For this review, take the finished solid that the model builds, in its own axes (mm). Face numbers are marked on the shaded views. A direction names the side the tool comes from. Coordinates: 2 decimals unless noted, no trailing zeros. Loops run counter-clockwise (first coordinate to the right, second up) from the corner with the lowest first, then second, coordinate; pieces in that order, holes last. Notation, with made-up numbers: (-4, 65) - (47, 65) arc R25 ccw to (47, 84) - close; hole circle Ø6 at (-17, 26.25). An arc over 180 degrees is marked (long way). Use one line per item in the form item = value. Start each with the question number.
1. Add section A-A on z = -35. Give the boundary of the cut face in (x, y).
2. For pin 1 Ø10 at (x, y) = (124.5, -20) entering from -Z; pin 2 Ø12.5 at (y, z) = (-15, 22) entering from +X; pin 3 Ø7.5 at (x, y) = (20.5, -8.5) entering from +Z; pin 4 Ø8 at (x, y) = (-37.5, -15.5) entering from +Z, all flat-tipped, find the tip position at first contact; note any pin that passes through.
3. Draft analysis for pull direction X (two halves, no side actions). For the marked faces 5, 6, 7 and 8, state which applies: +X half, -X half, draft (parallel to the pull), parting line (faces both ways), or undercut.
4. Add section C-C on z = -5. Give the boundary of the cut face in (x, y), and give its area (3 significant figures).
5. Add section B-B on x = 86. Give the boundary of the cut face in (y, z).
6. Add section D-D on z = -20.5. Give the boundary of the cut face in (x, y).
7. To check wall thickness, follow probe 1 along Z at (x, y) = (76, -8.5); probe 2 along X at (y, z) = (-11.5, -5.5); probe 3 along X at (y, z) = (-5.5, -26). State the ranges of each line that lie inside material, in increasing order.
8. Machinability: for the marked faces 1, 2, 3 and 4, which of the approach directions +Z, -Z, +X, -X, +Y, -Y give a long, thin tool a straight path to every point of the face, cutting with its end or side? Answer none if there is none.
```python
from build123d import *

# Parameters (mm, degrees)
F1_DEPTH = 25.4


with BuildPart() as f1:
    # F0 (on Front) → F1 (new body)
    with BuildSketch(Plane.XZ):
        Polygon((-58.56847018, 26.8058441579), (-58.56847018, 44.1696718335), (-75.8564463832, 44.1696718335), (-87.0612412691, 22.8805579245), (-98.826281338, 44.1696718335), (-116.1657199264, 44.1696718335), (-116.1657199264, -44.1696718335), (-97.4510317668, -44.1696718335), (-97.4510317668, 8.7780756876), (-87.0612412691, -2.158543095), (-75.5490139127, 8.7780756876), (-75.5490139127, -44.1696718335), (-58.56847018, -44.1696718335), align=None)
        Polygon((-7.5672003441, 26.8058441579), (-7.5672003441, 44.1696718335), (-16.0395050349, 44.1696718335), (-32.1926623583, 26.0362979025), (-50.0853913032, 44.1696718335), (-58.56847018, 44.1696718335), (-58.56847018, 26.8058441579), (-41.1093979278, 9.8758367822), (-41.1093979278, -44.1696718335), (-23.9841751754, -44.1696718335), (-23.9841751754, 9.8758367822), align=None)
        Polygon((9.3628074974, -29.6275112778), (9.3628074974, 44.1696718335), (-7.5672003441, 44.1696718335), (-7.5672003441, 26.8058441579), (-7.5672003441, -44.1696718335), (40.4011495411, -44.1696718335), (40.4011495411, -29.6275112778), align=None)
        Polygon((116.1657199264, 44.110127064), (116.1657199264, 44.1696718335), (40.4011495411, 44.1696718335), (40.4011495411, -29.6275112778), (40.4011495411, -44.1696718335), (116.1657199264, -44.1696718335), (116.1657199264, -44.110127064), (100.1692116261, -44.110127064), (100.1692116261, -25.7797837257), (63.4875297546, -25.7797837257), (63.4875297546, 5.258561112), (79.1349560022, 5.258561112), (79.1349560022, 15.0061408058), (63.4875297546, 15.0061408058), (63.4875297546, 26.5493281186), (100.1692116261, 26.5493281186), (100.1692116261, 44.110127064), align=None)
        Polygon((157.1156084538, 44.110127064), (116.1657199264, 44.110127064), (116.1657199264, -10.1323537529), (135.5683207512, -10.1323537529), (135.5683207512, -26.8058460206), (121.2034597993, -26.8058460206), (121.2034597993, -12.4409906566), (116.1657199264, -12.4409906566), (116.1657199264, -44.110127064), (157.1156084538, -44.110127064), (157.1156084538, 7.054167334), (119.920887053, 7.054167334), (119.920887053, 23.21462892), (157.1156084538, 23.21462892), align=None)
        Polygon((116.1657199264, -10.1323537529), (116.1657199264, 44.110127064), (100.1692116261, 44.110127064), (100.1692116261, 26.5493281186), (100.1692116261, -10.1323537529), align=None)
        Polygon((116.1657199264, -44.110127064), (116.1657199264, -12.4409906566), (100.1692116261, -12.4409906566), (100.1692116261, -25.7797837257), (100.1692116261, -44.110127064), align=None)
    extrude(amount=F1_DEPTH)


solid = f1.part
```
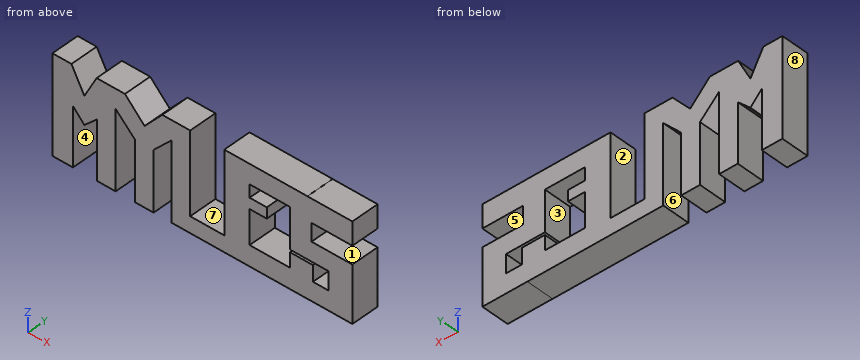
Conclusion:
q1.outline = (-116.17, -25.4) - (-97.45, -25.4) - (-97.45, 0) - (-116.17, 0) - close; (-75.55, -25.4) - (-58.57, -25.4) - (-58.57, 0) - (-75.55, 0) - close; (-41.11, -25.4) - (-23.98, -25.4) - (-23.98, 0) - (-41.11, 0) - close; (-7.57, -25.4) - (157.12, -25.4) - (157.12, 0) - (-7.57, 0) - close
q2.pin_1 = -44.11
q2.pin_2 = 157.12
q2.pin_3 = -29.63
q2.pin_4 = 35.47
q3.face_5 = draft
q3.face_6 = undercut
q3.face_7 = undercut
q3.face_8 = -X half
q4.outline = (-116.17, -25.4) - (-97.45, -25.4) - (-97.45, 0) - (-116.17, 0) - close; (-75.55, -25.4) - (-58.57, -25.4) - (-58.57, 0) - (-75.55, 0) - close; (-41.11, -25.4) - (-23.98, -25.4) - (-23.98, 0) - (-41.11, 0) - close; (-7.57, -25.4) - (9.36, -25.4) - (9.36, 0) - (-7.57, 0) - close; (40.4, -25.4) - (63.49, -25.4) - (63.49, 0) - (40.4, 0) - close; (100.17, -25.4) - (157.12, -25.4) - (157.12, 0) - (100.17, 0) - close
q4.area = 3,800 mm^2
q5.outline = (-25.4, -44.17) - (0, -44.17) - (0, -25.78) - (-25.4, -25.78) - close; (-25.4, 26.55) - (0, 26.55) - (0, 44.17) - (-25.4, 44.17) - close
q6.outline = (-116.17, -25.4) - (-97.45, -25.4) - (-97.45, 0) - (-116.17, 0) - close; (-75.55, -25.4) - (-58.57, -25.4) - (-58.57, 0) - (-75.55, 0) - close; (-41.11, -25.4) - (-23.98, -25.4) - (-23.98, 0) - (-41.11, 0) - close; (-7.57, -25.4) - (9.36, -25.4) - (9.36, 0) - (-7.57, 0) - close; (40.4, -25.4) - (63.49, -25.4) - (63.49, 0) - (40.4, 0) - close; (100.17, -25.4) - (121.2, -25.4) - (121.2, 0) - (100.17, 0) - close; (135.57, -25.4) - (157.12, -25.4) - (157.12, 0) - (135.57, 0) - close
q7.probe_1 = -44.17 to -25.78, 5.26 to 15.01, 26.55 to 44.17
q7.probe_2 = -116.17 to -97.45, -75.55 to -58.57, -41.11 to -23.98, -7.57 to 9.36, 40.4 to 63.49, 100.17 to 157.12
q7.probe_3 = -116.17 to -97.45, -75.55 to -58.57, -41.11 to -23.98, -7.57 to 9.36, 40.4 to 121.2, 135.57 to 157.12
q8.face_1 = +X, +Y, -Y
q8.face_2 = +Z, +Y, -Y
q8.face_3 = +Y, -Y
q8.face_4 = -Z, +Y, -Y
